Geometry: final body of the model. Coordinates: model frame, mm. Face numbers are marked on the shaded views. A direction names the side the tool comes from. Round coordinates to 2 decimals unless told otherwise and drop trailing zeros. Loops run counter-clockwise (first coordinate to the right, second up) from the corner with the lowest first, then second, coordinate; pieces in that order, holes last. Notation, with made-up numbers: M 19,-10.5 L 58,-10.5 A11 cw 58,-5.5 Z; hole C 33,66 d8. An arc over 180 degrees is marked long. Answer as a JSON object with one key per item and string values.
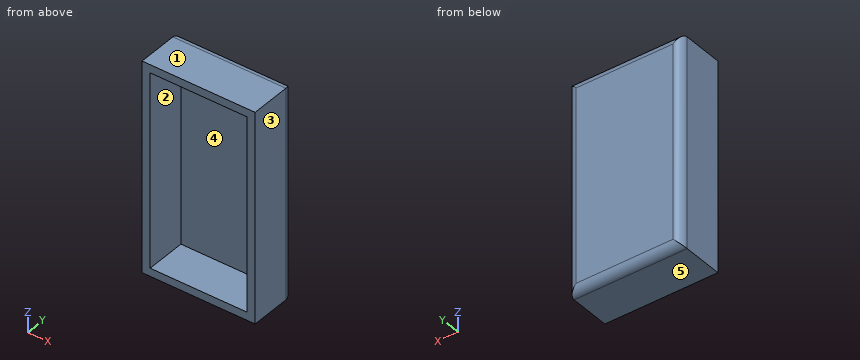
from build123d import *

# Parameters (mm, degrees)
F0_W     = 35
F0_H     = 65
F1_DEPTH = 15
F2_T     = -2.5
F3_R     = 2.5


with BuildPart() as f1:
    # F0 (on Front) → F1 (new body)
    with BuildSketch(Plane.XZ):
        with Locations((17.5, 32.5)):
            Rectangle(F0_W, F0_H)
    extrude(amount=F1_DEPTH)

    # F2
    f2_openings = [f1.faces().sort_by_distance(p)[0] for p in [
        (17.5, -15, 32.5),
    ]]
    offset(amount=F2_T, openings=f2_openings)

    # F3
    f3_edges = [f1.edges().sort_by_distance(p)[0] for p in [
        (0, 0, 32.5),
        (17.5, 0, 0),
        (35, 0, 32.5),
        (17.5, 0, 65),
    ]]
    fillet(f3_edges, radius=F3_R)


solid = f1.part
1) Section query A-A (y = -10.75). Return the cut outline in (x, z).
Results:
{"outline": "M 0,0 L 35,0 L 35,65 L 0,65 Z; hole M 2.5,2.5 L 32.5,2.5 L 32.5,62.5 L 2.5,62.5 Z"}
2) Section query B-B (z = 53.5). Return the cut outline in (x, y).
Results:
{"outline": "M 0,-15 L 2.5,-15 L 2.5,-2.5 L 32.5,-2.5 L 32.5,-15 L 35,-15 L 35,-2.5 A2.5 ccw 32.5,0 L 2.5,0 A2.5 ccw 0,-2.5 Z"}
3) Section query C-C (x = 21.5). Return the cut outline in (y, z), and give its area (3 significant figures).
Results:
{"outline": "M -15,0 L -2.5,0 A2.5 ccw 0,2.5 L 0,62.5 A2.5 ccw -2.5,65 L -15,65 L -15,62.5 L -2.5,62.5 L -2.5,2.5 L -15,2.5 Z", "area": "222 mm2"}
4) Pull-direction query (Z, two-part tool) for the marked faces 1, 2 and 3; classes: +Z half, -Z half, draft (parallel to the pull), parting line (faces both ways), or undercut.
Results:
{"face 1": "+Z half", "face 2": "undercut", "face 3": "draft"}
5) Reachability of the marked faces 4 and 5 from +Z, -Z, +X, -X, +Y, -Y: full face, straight path, thin tool, end or side. Return the list, or none.
Results:
{"face 4": "-Y", "face 5": "-Z, +X, -X, +Y, -Y"}
6) Pin query (flat end, axial travel): P1, Ø6, axis at y = -2, z = 10, coming from the +X side; P2, Ø15, axis at x = 21.5, z = 30.5, coming from the -Y side. Return the tip coordinate at first contact, or that it passes through.
Results:
{"P1": "x = 35", "P2": "y = -2.5"}
7) Ray query, line 1 (X direction, y = -6.25, z = 5); line 2 (Z direction, x = 30, y = -3); line 3 (Y direction, x = 30, z = 43). Return the intervals inside material, ascending.
Results:
{"line 1": "0 to 2.5, 32.5 to 35", "line 2": "0 to 2.5, 62.5 to 65", "line 3": "-2.5 to 0"}
